Design review of the part built by this model. Coordinates are the model's own, in mm. Give positions to 0.01 mm unless a question says otherwise; leave off trailing zeros. Write each loop counter-clockwise with the first axis right and the second up, starting at its lowest first coordinate (ties: lowest second). Pieces come first, ordered by that corner, then holes.
```python
from build123d import *

# Parameters (mm, degrees)
SKETCH_1_W          = 140
SKETCH_1_H          = 103
EXTRUDE_1_DEPTH     = 3
SKETCH_2_R          = 1.5
SKETCH_2_R_2        = 1.55
CUT_EXTRUDE_1_DEPTH = 87.955448363


with BuildPart() as part:
    # 草图1 → 凸台-拉伸1 (new body)
    with BuildSketch(Plane.XY):
        Rectangle(SKETCH_1_W, SKETCH_1_H)
    extrude(amount=EXTRUDE_1_DEPTH)

    # 草图2 → 切除-拉伸1 (cut, through all)
    with BuildSketch(Plane.XY.offset(3)):
        with Locations((-60, 26.5)):
            Circle(SKETCH_2_R)
        with Locations((60, 26.5)):
            Circle(SKETCH_2_R_2)
        with Locations((0, -38.5)):
            Circle(SKETCH_2_R_2)
    extrude(amount=-CUT_EXTRUDE_1_DEPTH, mode=Mode.SUBTRACT)


solid = part.part
```
(1) Mouldability with a two-part tool opening along Y and no side actions: class faces 1 (the face through (-1, 51.5, 1)), 2 (the face through (-1, -51.5, 1)), 3 (the face through (-0.336, -40.013, 1.521)) as pulls with the +Y half, pulls with the -Y half, needs draft (parallel to the pull), parting line crosses it, or undercut.
Resolved:
face 1: pulls with the +Y half
face 2: pulls with the -Y half
face 3: undercut
(2) To check wall thickness, follow L1, parallel to Y at x = 60, z = 1; L2, parallel to Y at x = 0, z = 1.8; L3, parallel to X at y = -39, z = 2.5. State the ranges of each line that lie inside material, in increasing order.
Resolved:
L1: y = -51.5 to 24.95, 28.05 to 51.5
L2: y = -51.5 to -40.05, -36.95 to 51.5
L3: x = -70 to -1.47, 1.47 to 70
(3) Consider section B-B, the plane x = 0. Give the boundary of the cut face in (y, z), then the cut area to 3 significant figures.
Resolved:
outline: (-51.5, 0) - (-40.05, 0) - (-40.05, 3) - (-51.5, 3) - close; (-36.95, 0) - (51.5, 0) - (51.5, 3) - (-36.95, 3) - close
area: 300 mm2
(4) Consider section A-A, the plane x = -60. Give the boundary of the cut face in (y, z), then the cut area to 3 significant figures.
Resolved:
outline: (-51.5, 0) - (25, 0) - (25, 3) - (-51.5, 3) - close; (28, 0) - (51.5, 0) - (51.5, 3) - (28, 3) - close
area: 300 mm2
